Build history of the part. All positions in model axes, mm. A direction names the side the tool comes from. Round coordinates to 2 decimals unless told otherwise and drop trailing zeros. Order: outer loops, then holes, each group sorted by start corner. A loop starts at its lowest first (then second) coordinate and runs counter-clockwise, first axis right, second up. Notation, with made-up numbers: (-13, 89.25) -> (34, 89.25) arc R23 cw to (34, 120.25) -> close; hole circle Ø8 at (81.25, 33). An arc over 180 degrees is marked (long way). Use a Markdown table: item, result. Add a question column.
Item 1: Pin check, flat tips, straight feed: pin 1 (5 mm diameter, centred on y = 1, z = -16.5, fed in from +X); pin 2 (0.6 mm diameter, centred on x = -0.5, y = -1.5, fed in from +Z); pin 3 (1 mm diameter, centred on y = -1.5, z = -10, fed in from -X). Stop position of each tip, or through.
Item 2: Slice it at A-A, the plane z = -17.5. Give the cut face in (x, y), plus the area to 3 significant figures.
Item 3: Two-plate mould, pull along X, no slides. Class faces 4 (the face through (-2.32, -0.58, 3.77)), 5 (the face through (0, 0, -30)), 6 (the face through (2.285, -3.584, 2.469)): released by +X, released by -X, zero draft, split by the parting line, or undercut.
Item 4: Probe L1, parallel to Z at x = 3.5, y = -0.5; L2, parallel to Z at x = -1.5, y = 1.25; L3, parallel to Y at x = -1.5, z = -13. List the from-to ranges inside material, lowest first.
Item 5: 3-axis set-ups, long thin cutter, end or side, ignore diameter. For faces 1 (the face through (1, -3, 0)), 2 (the face through (2, -2, 5)), 3 (the face through (1.663, -1.719, 3.768)): which of +Z, -Z, +X, -X, +Y, -Y reach the whole face in a straight line?
Solid Edge part; units mm, degrees
sketch "Sketch1" plane through (0, 0, 0) normal (0, -1, 0) x (1, 0, 0)
  line L0 (4.25, 5) -> (4.25, 0)
  line L1 (4.25, 0) -> (2.85, 0)
  line L2 (2.85, 0) -> (2.5, -0.6062)
  line L3 (2.5, -0.6062) -> (2.5, -30)
  line L4 (2.5, -30) -> (0, -30)
  line L5 (2.3, 2.5) -> (0, 1.1721)
  line L6 (2.3, 5) -> (2.3, 2.5)
  line L7 (4.25, 5) -> (2.3, 5)
revolve "RevolvedProtrusion1" add sketch "Sketch1" angle 360 about axis through (0, 0, -6) along (0, 0, 1)
cosmetic_thread "Thread1"
chamfer "Chamfer_1" distance 0.25 angle 45 1 edges at (-2.5, 0, -30)
fillet "Round_1" radius 0.3 2 edges at (-4.25, 0, 0) (-4.25, 0, 5)
sketch "Sketch2" plane through (0, 0, 5) normal (0, 0, 1) x (0, 1, 0)
  line L0 (-2.3, 1.3279) -> (-2.3, -1.3279)
  line L1 (0, -2.6558) -> (-2.3, -1.3279)
  line L2 (2.3, -1.3279) -> (0, -2.6558)
  line L3 (2.3, 1.3279) -> (2.3, -1.3279)
  line L4 (0, 2.6558) -> (2.3, 1.3279)
  line L5 (-2.3, 1.3279) -> (0, 2.6558)
extrude "Cutout1" cut sketch "Sketch2" against normal up to vertex (2.5 mm away)
properties material "Galvanized steel"
Check sheet entries:
| question | item | result |
|---|---|---|
| 1 | pin 1 | x = 2.5 |
| 1 | pin 2 | z = 2.26 |
| 1 | pin 3 | x = -2.29 |
| 2 | outline | circle Ø5 at (0, 0) |
| 2 | area | 19.6 mm2 |
| 3 | face 4 | undercut |
| 3 | face 5 | zero draft |
| 3 | face 6 | split by the parting line |
| 4 | L1 | 0 to 5 |
| 4 | L2 | -30 to 2.3 |
| 4 | L3 | -2 to 2 |
| 5 | face 1 | -Z |
| 5 | face 2 | +Z, +X, -X, +Y, -Y |
| 5 | face 3 | +Z |
